```python
from build123d import *

# Parameters (mm, degrees)
SKETCH1_R           = 21.5
SKETCH1_R_2         = 15.5
SKETCH1_R_3         = 1.5
BOSS_EXTRUDE1_DEPTH = 3
SKETCH2_R           = 2.5
BOSS_EXTRUDE2_DEPTH = 29
SKETCH3_R           = 1.5
CUT_EXTRUDE1_DEPTH  = 5


with BuildPart() as part:
    # Sketch1 → Boss-Extrude1 (new body)
    with BuildSketch(Plane(origin=(0, 0, 0), x_dir=(1, 0, 0), z_dir=(0, 1, 0))):
        with Locations(Location((0, 0, 0), (0, 0, 270))):
            Circle(SKETCH1_R)
        with Locations(Location((0, 0, 0), (0, 0, 270))):
            Circle(SKETCH1_R_2, mode=Mode.SUBTRACT)
        with Locations(Location((0, 18.5, 0), (0, 0, 270))):
            Circle(SKETCH1_R_3, mode=Mode.SUBTRACT)
        with Locations(Location((18.5, 0, 0), (0, 0, 270))):
            Circle(SKETCH1_R_3, mode=Mode.SUBTRACT)
        with Locations(Location((0, -18.5, 0), (0, 0, 270))):
            Circle(SKETCH1_R_3, mode=Mode.SUBTRACT)
        with Locations(Location((-18.5, 0, 0), (0, 0, 270))):
            Circle(SKETCH1_R_3, mode=Mode.SUBTRACT)
    extrude(amount=BOSS_EXTRUDE1_DEPTH)

    # Sketch2 → Boss-Extrude2 (add)
    with BuildSketch(Plane(origin=(0, 3, 0), x_dir=(1, 0, 0), z_dir=(0, 1, 0))):
        with Locations(Location((-13.081475452, 13.081475452, 0), (0, 0, 90))):
            Circle(SKETCH2_R)
        with Locations(Location((13.081475452, 13.081475452, 0), (0, 0, 90))):
            Circle(SKETCH2_R)
        with Locations(Location((13.081475452, -13.081475452, 0), (0, 0, 90))):
            Circle(SKETCH2_R)
        with Locations(Location((-13.081475452, -13.081475452, 0), (0, 0, 90))):
            Circle(SKETCH2_R)
    extrude(amount=BOSS_EXTRUDE2_DEPTH)

    # Sketch3 → Cut-Extrude1 (cut)
    with BuildSketch(Plane(origin=(0, 32, 0), x_dir=(1, 0, 0), z_dir=(0, 1, 0))):
        with Locations(Location((-13.081475452, 13.081475452, 0), (0, 0, 270))):
            Circle(SKETCH3_R)
        with Locations(Location((13.081475452, 13.081475452, 0), (0, 0, 270))):
            Circle(SKETCH3_R)
        with Locations(Location((13.081475452, -13.081475452, 0), (0, 0, 270))):
            Circle(SKETCH3_R)
        with Locations(Location((-13.081475452, -13.081475452, 0), (0, 0, 270))):
            Circle(SKETCH3_R)
    extrude(amount=-CUT_EXTRUDE1_DEPTH, mode=Mode.SUBTRACT)


solid = part.part
```
For this review, take the finished solid that the model builds, in its own axes (mm). A direction names the side the tool comes from. Round coordinates to 2 decimals unless told otherwise and drop trailing zeros. Order: outer loops, then holes, each group sorted by start corner. A loop starts at its lowest first (then second) coordinate and runs counter-clockwise, first axis right, second up.
Q1. Machinability: for faces 1 (the flat face through (13, 32, -15)), 2 (the cylindrical face through (12.331, 17.297, -15.466)), which of the approach directions +Z, -Z, +X, -X, +Y, -Y give a long, thin tool a straight path to every point of the face, cutting with its end or side? Answer none if there is none.
Findings below:
face 1: +Z, -Z, +X, -X, +Y
face 2: +Y
Q2. We need section D-D, the plane y = 24. Give the boundary of the cut face in (x, z), plus the area to 3 significant figures.
Findings below:
outline: circle Ø5 at (-13.08, -13.08); circle Ø5 at (-13.08, 13.08); circle Ø5 at (13.08, -13.08); circle Ø5 at (13.08, 13.08)
area: 78.5 mm2
Q3. Mouldability with a two-part tool opening along X and no side actions: class faces 3 (the cylindrical face through (14.531, 1.479, -15.846)), 4 (the flat face through (-13, 32, 11)), 5 (the cylindrical face through (0, 1, 17)) as pulls with the +X half, pulls with the -X half, needs draft (parallel to the pull), parting line crosses it, or undercut.
Findings below:
face 3: parting line crosses it
face 4: needs draft
face 5: undercut
Q4. Insertion check: P1, Ø0.9, axis at x = 13, z = -13, coming from the +Y side; P2, Ø25, axis at x = 0, z = 0, coming from the +Y side; P3, Ø5, axis at x = -18.5, z = 0, coming from the +Y side; P4, Ø1, axis at y = 22.5, z = -12.5, coming from the -X side. Each pin has a flat end and moves straight along its axis. Give the tip position at first contact, or say it passes through.
Findings below:
P1: stops at y = 27
P2: passes through
P3: stops at y = 3
P4: stops at x = -15.58
Q5. Wall thickness on line 1 (X direction, y = 1.7, z = 0); line 2 (Y direction, x = 3, z = 16); line 3 (Z direction, x = -15, y = 9.5): over which ranges is each line inside the solid? List them lowest first.
Findings below:
line 1: x = -21.5 to -20, -17 to -15.5, 15.5 to 17, 20 to 21.5
line 2: y = 0 to 3
line 3: z = -14.68 to -11.48, 11.48 to 14.68
Q6. We need section A-A, the plane z = 0. Give the boundary of the cut face in (x, y), plus the area to 3 significant figures.
Findings below:
outline: (-21.5, 0) - (-20, 0) - (-20, 3) - (-21.5, 3) - close; (-17, 0) - (-15.5, 0) - (-15.5, 3) - (-17, 3) - close; (15.5, 0) - (17, 0) - (17, 3) - (15.5, 3) - close; (20, 0) - (21.5, 0) - (21.5, 3) - (20, 3) - close
area: 18.0 mm2
Q7. We need section C-C, the plane z = 12.5. Give the boundary of the cut face in (x, y).
Findings below:
outline: (-17.49, 0) - (-9.17, 0) - (-9.17, 3) - (-10.65, 3) - (-10.65, 32) - (-11.7, 32) - (-11.7, 27) - (-14.46, 27) - (-14.46, 32) - (-15.51, 32) - (-15.51, 3) - (-17.49, 3) - close; (9.17, 0) - (17.49, 0) - (17.49, 3) - (15.51, 3) - (15.51, 32) - (14.46, 32) - (14.46, 27) - (11.7, 27) - (11.7, 32) - (10.65, 32) - (10.65, 3) - (9.17, 3) - close
Q8. We need section B-B, the plane x = 8. Give the boundary of the cut face in (y, z), plus the area to 3 significant figures.
Findings below:
outline: (0, -19.96) - (3, -19.96) - (3, -13.28) - (0, -13.28) - close; (0, 13.28) - (3, 13.28) - (3, 19.96) - (0, 19.96) - close
area: 40.1 mm2
